Could you check a few things on this model? Use its own coordinates, in mm. A direction names the side the tool comes from. Round coordinates to 2 decimals unless told otherwise and drop trailing zeros. Loops run counter-clockwise (first coordinate to the right, second up) from the corner with the lowest first, then second, coordinate; pieces in that order, holes last. Notation, with made-up numbers: (28.5, 28) -> (42.5, 28) arc R28 ccw to (42.5, 52) -> close; hole circle Ø6 at (-17.5, 34). An arc over 180 degrees is marked (long way). One line per item, written item: value.
```python
from build123d import *

# Parameters (mm, degrees)
F0_R      = 15.433167194
F0_R_2    = 8.0548322191
F1_DEPTH  = 25.4
F2_W      = 17.1370897226
F2_H      = 13.9400362968
F3_DEPTH  = 52.07
F4_W      = 17.1583444834
F4_H      = 14.7807182949
F5_DEPTH  = 100.076
F7_W      = 20.3292299993
F7_H      = 28.4609068185
F8_DEPTH  = 57.658
F9_W      = 20.3302133896
F9_H      = 28.3219206433
F10_DEPTH = 54.61
F11_W     = 19.8471819321
F11_H     = 48.8284118474
F11_W_2   = 19.9860688299
F11_H_2   = 48.6484020948
F12_DEPTH = 44.704
F13_R     = 29.6448056137
F13_R_2   = 17.9422846096
F14_DEPTH = 21.082
F15_R     = 19.0161777789
F15_R_2   = 7.7492998165
F16_DEPTH = 31.242


with BuildPart() as f1:
    # F0 (on Front) → F1 (new body)
    with BuildSketch(Plane.XZ):
        Polygon((19.0223418176, 28.2409206692), (19.0223418176, 59.6059984693), (9.2501137406, 59.6059984693), (-9.0077609013, 59.6059984693), (-18.3395408094, 59.6059984693), (-18.3395408094, 28.2409206692), (-9.0077609013, 28.2409206692), (9.2501137406, 28.2409206692), align=None)
        with Locations((0.1452074648, 43.853033334)):
            Circle(F0_R, mode=Mode.SUBTRACT)
        with BuildLine():
            Line((9.2501137406, -37.7542672334), (9.2501137406, 15.5216934006))
            ThreePointArc((9.2501137406, 15.5216934006), (0.1272952852, 14.0501270571), (-9.0077609013, 15.4437096852))
            Line((-9.0077609013, 15.4437096852), (-9.0077609013, -37.7542672334))
            Line((-9.0077609013, -37.7542672334), (9.2501137406, -37.7542672334))
        make_face()
        with Locations((0.1452074648, 43.853033334)):
            Circle(F0_R)
        with Locations((0, 43.853033334)):
            Circle(F0_R_2, mode=Mode.SUBTRACT)
        with BuildLine():
            Line((19.0223418176, -37.7542672334), (19.0223418176, 20.9100618958))
            ThreePointArc((19.0223418176, 20.9100618958), (14.3906763073, 17.7544153235), (9.2501137406, 15.5216934006))
            Line((9.2501137406, 15.5216934006), (9.2501137406, -37.7542672334))
            Line((9.2501137406, -37.7542672334), (19.0223418176, -37.7542672334))
        make_face()
        with BuildLine():
            Line((-9.0077609013, -37.7542672334), (-9.0077609013, 15.4437096852))
            ThreePointArc((-9.0077609013, 15.4437096852), (-13.8929074263, 17.4860738983), (-18.3395408094, 20.360679907))
            Line((-18.3395408094, 20.360679907), (-18.3395408094, -37.7542672334))
            Line((-18.3395408094, -37.7542672334), (-9.0077609013, -37.7542672334))
        make_face()
        with BuildLine():
            Line((-18.3395408094, 59.6059984693), (-18.3395408094, 67.345386761))
            ThreePointArc((-18.3395408094, 67.345386761), (-29.8031781298, 43.853033334), (-18.3395408094, 20.360679907))
            Line((-18.3395408094, 20.360679907), (-18.3395408094, 28.2409206692))
            Line((-18.3395408094, 28.2409206692), (-18.3395408094, 59.6059984693))
        make_face()
        with BuildLine():
            ThreePointArc((19.0223418176, 20.9100618958), (26.973650738, 31.178192408), (29.8031781298, 43.853033334))
            ThreePointArc((29.8031781298, 43.853033334), (26.973650738, 56.5278742601), (19.0223418176, 66.7960047722))
            Line((19.0223418176, 66.7960047722), (19.0223418176, 59.6059984693))
            Line((19.0223418176, 59.6059984693), (19.0223418176, 28.2409206692))
            Line((19.0223418176, 28.2409206692), (19.0223418176, 20.9100618958))
        make_face()
        with BuildLine():
            ThreePointArc((-9.0077609013, 15.4437096852), (0.1272952852, 14.0501270571), (9.2501137406, 15.5216934006))
            Line((9.2501137406, 15.5216934006), (9.2501137406, 28.2409206692))
            Line((9.2501137406, 28.2409206692), (-9.0077609013, 28.2409206692))
            Line((-9.0077609013, 28.2409206692), (-9.0077609013, 15.4437096852))
        make_face()
        with BuildLine():
            Line((9.2501137406, 59.6059984693), (9.2501137406, 72.1843732675))
            ThreePointArc((9.2501137406, 72.1843732675), (0.1272952852, 73.6559396109), (-9.0077609013, 72.2623569828))
            Line((-9.0077609013, 72.2623569828), (-9.0077609013, 59.6059984693))
            Line((-9.0077609013, 59.6059984693), (9.2501137406, 59.6059984693))
        make_face()
        with BuildLine():
            ThreePointArc((9.2501137406, 15.5216934006), (14.3906763073, 17.7544153235), (19.0223418176, 20.9100618958))
            Line((19.0223418176, 20.9100618958), (19.0223418176, 28.2409206692))
            Line((19.0223418176, 28.2409206692), (9.2501137406, 28.2409206692))
            Line((9.2501137406, 28.2409206692), (9.2501137406, 15.5216934006))
        make_face()
        with BuildLine():
            Line((19.0223418176, 59.6059984693), (19.0223418176, 66.7960047722))
            ThreePointArc((19.0223418176, 66.7960047722), (14.3906763073, 69.9516513445), (9.2501137406, 72.1843732675))
            Line((9.2501137406, 72.1843732675), (9.2501137406, 59.6059984693))
            Line((9.2501137406, 59.6059984693), (19.0223418176, 59.6059984693))
        make_face()
        with BuildLine():
            ThreePointArc((-18.3395408094, 20.360679907), (-13.8929074263, 17.4860738983), (-9.0077609013, 15.4437096852))
            Line((-9.0077609013, 15.4437096852), (-9.0077609013, 28.2409206692))
            Line((-9.0077609013, 28.2409206692), (-18.3395408094, 28.2409206692))
            Line((-18.3395408094, 28.2409206692), (-18.3395408094, 20.360679907))
        make_face()
        with BuildLine():
            Line((-9.0077609013, 59.6059984693), (-9.0077609013, 72.2623569828))
            ThreePointArc((-9.0077609013, 72.2623569828), (-13.8929074263, 70.2199927697), (-18.3395408094, 67.345386761))
            Line((-18.3395408094, 67.345386761), (-18.3395408094, 59.6059984693))
            Line((-18.3395408094, 59.6059984693), (-9.0077609013, 59.6059984693))
        make_face()
    extrude(amount=F1_DEPTH)

    # F2 (on Top) → F3 (cut)
    with BuildSketch(Plane.XY):
        with Locations((-0.8700220022, -19.4579679519)):
            Rectangle(F2_W, F2_H)
    extrude(amount=-F3_DEPTH, mode=Mode.SUBTRACT)

    # F4 (on Top) → F5 (cut)
    with BuildSketch(Plane.XY):
        with Locations((-0.8593946218, -19.5878909072)):
            Rectangle(F4_W, F4_H)
    extrude(amount=F5_DEPTH, mode=Mode.SUBTRACT)

    # F7 (on Right) → F8 (cut)
    with BuildSketch(Plane.YZ):
        with Locations((-17.8606694099, 44.7242846712)):
            Rectangle(F7_W, F7_H)
    extrude(amount=F8_DEPTH, mode=Mode.SUBTRACT)

    # F9 (on Right) → F10 (cut)
    with BuildSketch(Plane.YZ):
        with Locations((-17.5707505118, 44.6547915836)):
            Rectangle(F9_W, F9_H)
    extrude(amount=-F10_DEPTH, mode=Mode.SUBTRACT)

    # F11 (on Front) → F12 (cut)
    with BuildSketch(Plane.XZ):
        with Locations((29.1418134246, 44.8984373361)):
            Rectangle(F11_W, F11_H)
        with Locations((-28.1968573108, 44.9884422123)):
            Rectangle(F11_W_2, F11_H_2)
    extrude(amount=F12_DEPTH, mode=Mode.SUBTRACT)

    # F13 (on face) → F14 (join)
    with BuildSketch(Plane.XZ):
        with Locations((0, 43.9448542893)):
            Circle(F13_R)
        with Locations((0, 43.9448542893)):
            Circle(F13_R_2, mode=Mode.SUBTRACT)
        with Locations((0, 43.9448542893)):
            Circle(F13_R_2)
        with BuildLine():
            ThreePointArc((-7.4182733413, 41.6264460763), (-1.1726275703, 51.6280008186), (7.772116572, 43.9448542893))
            ThreePointArc((7.772116572, 43.9448542893), (7.6831465293, 42.772226719), (7.4182733413, 41.6264460763))
            ThreePointArc((7.4182733413, 41.6264460763), (0, 36.1078109239), (-7.4182733413, 41.6264460763))
        make_face(mode=Mode.SUBTRACT)
    extrude(amount=-F14_DEPTH)

    # F15 (on face) → F16 (join)
    with BuildSketch(Plane(origin=(0, 21.082, 0), x_dir=(-1, 0, 0), z_dir=(0, 1, 0))):
        with Locations((0, 43.9448542893)):
            Circle(F15_R)
        with Locations((0, 43.9448542893)):
            Circle(F15_R_2, mode=Mode.SUBTRACT)
    extrude(amount=F16_DEPTH)


solid = f1.part
```
Item 1: If we section it at B-B on z = 4: List the corners of the cut face in (x, y) for me, plus the area to 3 significant figures.
Output:
outline: (-18.34, -25.4) -> (-9.44, -25.4) -> (-9.44, -12.2) -> (7.72, -12.2) -> (7.72, -25.4) -> (19.02, -25.4) -> (19.02, 0) -> (-18.34, 0) -> close
area: 722 mm²
Item 2: Will these pins go through, and if not, where does the flat tip stop? pin 1 Ø20.5 at (y, z) = (-19, 35.5) entering from +X; pin 2 Ø1 at (y, z) = (3, 46.5) entering from +X; pin 3 Ø4.5 at (x, z) = (-2.5, 67) entering from -Y.
Output:
pin 1: stops at x = 19.22
pin 2: stops at x = 29.57
pin 3: stops at y = -12.2
Item 3: If we section it at D-D on x = 11: List the corners of the cut face in (y, z) for me, plus the area to 3 significant figures.
Output:
outline: (-25.4, -37.75) -> (0, -37.75) -> (0, 16.42) -> (21.08, 16.42) -> (21.08, 28.43) -> (52.32, 28.43) -> (52.32, 59.46) -> (21.08, 59.46) -> (21.08, 71.47) -> (0, 71.47) -> (0, 71.55) -> (-25.4, 71.55) -> (-25.4, 58.95) -> (-7.7, 58.95) -> (-7.7, 30.49) -> (-25.4, 30.49) -> close
area: 4,400 mm²
Item 4: If we section it at C-C on y = 25.5: List the corners of the cut face in (x, z) for me, plus the area to 3 significant figures.
Output:
outline: circle Ø38.03 at (0, 43.94); hole circle Ø15.5 at (0, 43.94)
area: 947 mm²
Item 5: If we mould it in two halves opening along X, with no side actions, what happens to faces 3 (the face through (-18.204, -7, 44)), 4 (the face through (12, -15, 58.955)), 5 (the face through (19.218, -7, 44)), 6 (the face through (-1, -12.488, -19))? For each: released by +X, released by -X, zero draft, split by the parting line, or undercut.
Output:
face 3: released by -X
face 4: zero draft
face 5: released by +X
face 6: undercut
Item 6: I need wall thicknesses on line 1 (Z direction, x = 0, y = 16); line 2 (Z direction, x = 0, y = 39); line 3 (Y direction, x = -26, z = 36). Which ranges of each line are inside material? Lowest first, please. Write a range as from..to.
Output:
line 1: z = 14.3..36.11, 51.72..73.59
line 2: z = 24.93..36.2, 51.69..62.96
line 3: y = 0..21.08
Item 7: For faces 1 (the face through (-1, -12.198, 66)), 2 (the face through (-0.4, 21.082, 24.6)), which set-ups out of +Z, -Z, +X, -X, +Y, -Y let a thin tool reach every point of the face, with its end or its side?
Output:
face 1: +Z, -Y
face 2: +Y
